Geometry: final body of the model. Coordinates: model frame, mm. Face numbers are marked on the shaded views. A direction names the side the tool comes from. Round coordinates to 2 decimals unless told otherwise and drop trailing zeros. Loops run counter-clockwise (first coordinate to the right, second up) from the corner with the lowest first, then second, coordinate; pieces in that order, holes last. Notation, with made-up numbers: M 80.5,82 L 114.5,82 A14 cw 114.5,90 Z; hole C -31,19.25 d10. An arc over 180 degrees is marked long. Answer as a JSON object with one key per item and string values.
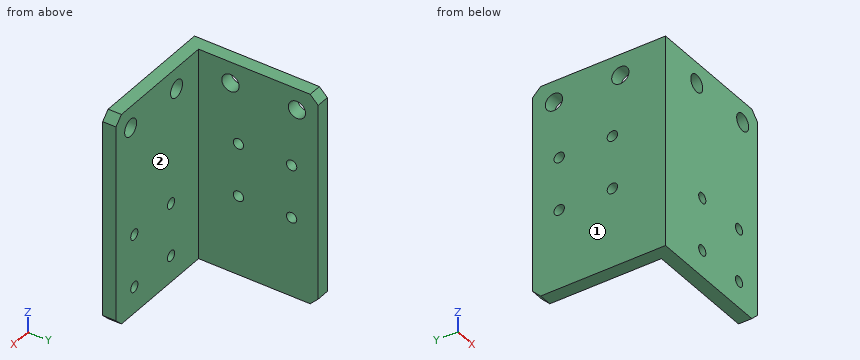
```python
from build123d import *

# Parameters (mm, degrees)
ESTRUSIONE_ESTRUSIONE1_DEPTH = 80
FORO_6_5_6_5_1_D             = 6.5
FORO_6_5_6_5_2_D             = 6.5
FORO_6_5_6_5_2_DEPTH         = 5
FORO_6_5_6_5_2_TIP           = 1.952797012
SMUSSO1_SIZE                 = 3
M3_5_CLEARANCE_HOLE1_D       = 3.9
M3_5_CLEARANCE_HOLE2_D       = 3.9


with BuildPart() as part:
    # Schizzo1 → Estrusione-Estrusione1 (new body)
    with BuildSketch(Plane.XY):
        Polygon((0, 0), (0, 50), (5, 50), (5, 5), (50, 5), (50, 0), align=None)
    extrude(amount=ESTRUSIONE_ESTRUSIONE1_DEPTH)

    # Foro Ø6.5 (6.5)-1 (through all)
    with Locations(Plane(origin=(0, 0, 0), x_dir=(-1, 0, 0), z_dir=(0, -1, 0))):
        with Locations((-17, -72), (-42, -72)):
            Hole(FORO_6_5_6_5_1_D / 2)

    # Foro Ø6.5 (6.5)-2
    with Locations(Plane.ZY):
        with Locations((72, 42), (72, 17)):
            Hole(FORO_6_5_6_5_2_D / 2, depth=FORO_6_5_6_5_2_DEPTH)
            with Locations((0, 0, -(FORO_6_5_6_5_2_DEPTH + FORO_6_5_6_5_2_TIP / 2))):  # 118° drill point
                Cone(0, FORO_6_5_6_5_2_D / 2, FORO_6_5_6_5_2_TIP, mode=Mode.SUBTRACT)

    # Smusso1
    smusso1_edges = [part.edges().sort_by_distance(p)[0] for p in [
        (2.5, 50, 80),
        (2.5, 50, 0),
        (50, 2.5, 80),
        (50, 2.5, 0),
    ]]
    chamfer(smusso1_edges, length=SMUSSO1_SIZE)

    # M3.5 Clearance Hole1 (through all)
    with Locations(Plane(origin=(20, 0, 30), x_dir=(-1, 0, 0), z_dir=(0, -1, 0))):
        with Locations((0, 0), (-20, 0), (-20, 20), (0, 20)):
            Hole(M3_5_CLEARANCE_HOLE1_D / 2)

    # M3.5 Clearance Hole2 (through all)
    with Locations(Plane(origin=(0, 40, 30), x_dir=(0, 0, -1), z_dir=(-1, 0, 0))):
        with Locations((0, 0), (-20, 0), (-20, 20), (0, 20)):
            Hole(M3_5_CLEARANCE_HOLE2_D / 2)


solid = part.part
```
1) Set-up query: the marked faces 1 and 2. Return all of +Z, -Z, +X, -X, +Y, -Y with unobstructed straight access to the full face (end or side cutting, diameter ignored); none if empty.
Geometry results:
{"face 1": "+Z, -Z, -X, +Y, -Y", "face 2": "+Z, -Z, +X, +Y"}
2) First-contact query: pin 1 (1 mm diameter, centred on x = 40.5, z = 25.5, fed in from +Y); pin 2 (4.5 mm diameter, centred on y = 40, z = 30, fed in from +X). Flat tips, straight axial feed; report the tip coordinate or a pass-through.
Geometry results:
{"pin 1": "y = 5", "pin 2": "x = 5"}
3) Line query: probe 1 along X at (y, z) = (1.7, 30); probe 2 along X at (y, z) = (4, 72); probe 3 along Z at (x, y) = (40, 3). Output: solid intervals per line, ascending.
Geometry results:
{"probe 1": "0 to 18.05, 21.95 to 38.05, 41.95 to 50", "probe 2": "0 to 13.75, 20.25 to 38.75, 45.25 to 50", "probe 3": "0 to 8.05, 11.95 to 28.05, 31.95 to 69.44, 74.56 to 80"}
4) Cut plane D-D on y = 23. Return the cut outline in (x, z), and give its area (3 significant figures).
Geometry results:
{"outline": "M 0,0 L 5,0 L 5,80 L 0,80 Z", "area": "400 mm2"}
5) Cut plane C-C on z = 72. Return the cut outline in (x, y), and give its area (3 significant figures).
Geometry results:
{"outline": "M 0,0 L 13.75,0 L 13.75,5 L 5,5 L 5,13.75 L 0,13.75 Z; M 0,20.25 L 5,20.25 L 5,38.75 L 0,38.75 Z; M 0,45.25 L 5,45.25 L 5,50 L 0,50 Z; M 20.25,0 L 38.75,0 L 38.75,5 L 20.25,5 Z; M 45.25,0 L 50,0 L 50,5 L 45.25,5 Z", "area": "345 mm2"}
6) Cut plane A-A on x = 17. Return the cut outline in (y, z), and give its area (4 significant figures).
Geometry results:
{"outline": "M 0,0 L 5,0 L 5,68.75 L 0,68.75 Z; M 0,75.25 L 5,75.25 L 5,80 L 0,80 Z", "area": "367.5 mm2"}
7) Cut plane B-B on z = 10. Return the cut outline in (x, y).
Geometry results:
{"outline": "M 0,0 L 18.05,0 L 18.05,5 L 5,5 L 5,50 L 0,50 Z; M 21.95,0 L 38.05,0 L 38.05,5 L 21.95,5 Z; M 41.95,0 L 50,0 L 50,5 L 41.95,5 Z"}
